```python
from build123d import *

# Parameters (mm, degrees)
SKETCH1_R            = 15
SKETCH1_R_2          = 1.25
BOSS_EXTRUDE1_DEPTH  = 1.3
FILLET1_R            = 1
SKETCH2_R            = 35.5
SKETCH2_R_2          = 0.625
BOSS_EXTRUDE2_DEPTH  = 0.1
SKETCH4_R            = 0.625
SKETCH4_R_2          = 31.5
BOSS_EXTRUDE4_DEPTH  = 0.1
SKETCH5_R            = 27.5
SKETCH5_R_2          = 0.625
BOSS_EXTRUDE5_DEPTH  = 0.1
SKETCH6_R            = 23.5
SKETCH6_R_2          = 0.625
BOSS_EXTRUDE6_DEPTH  = 0.1
SKETCH7_R            = 19.5
SKETCH7_R_2          = 0.625
BOSS_EXTRUDE7_DEPTH  = 0.1
SKETCH8_R            = 15.5
SKETCH8_R_2          = 0.625
BOSS_EXTRUDE8_DEPTH  = 0.1
BOSS_EXTRUDE9_DEPTH  = 0.1
BOSS_EXTRUDE10_DEPTH = 0.1
BOSS_EXTRUDE11_DEPTH = 0.1
BOSS_EXTRUDE12_DEPTH = 0.1
BOSS_EXTRUDE13_DEPTH = 0.1
BOSS_EXTRUDE14_DEPTH = 0.1
CUT_EXTRUDE1_START   = -1.5
SKETCH10_R           = 0.625
CUT_EXTRUDE1_DEPTH   = 1.5


with BuildPart() as part:
    # Sketch1 → Boss-Extrude1 (new body)
    with BuildSketch(Plane(origin=(0, 0, 0), x_dir=(1, 0, 0), z_dir=(0, 1, 0))):
        with BuildLine():
            ThreePointArc((-40, 0), (-29.325037044, -27.203716701), (-2.997889883, -39.8875))
            ThreePointArc((-2.997889883, -39.8875), (0, -43), (2.997889883, -39.8875))
            ThreePointArc((2.997889883, -39.8875), (40, 0), (2.997889883, 39.8875))
            ThreePointArc((2.997889883, 39.8875), (0, 43), (-2.997889883, 39.8875))
            ThreePointArc((-2.997889883, 39.8875), (-29.325037044, 27.203716701), (-40, 0))
        make_face()
        with Locations(Location((0, 0, 0), (0, 0, 270))):
            Circle(SKETCH1_R, mode=Mode.SUBTRACT)
        with Locations(Location((0, 40, 0), (0, 0, 270))):
            Circle(SKETCH1_R_2, mode=Mode.SUBTRACT)
        with Locations(Location((0, -40, 0), (0, 0, 270))):
            Circle(SKETCH1_R_2, mode=Mode.SUBTRACT)
    extrude(amount=BOSS_EXTRUDE1_DEPTH)

    # Fillet1
    fillet1_edges = [part.edges().sort_by_distance(p)[0] for p in [
        (-2.997889883, 0.65, -39.8875),
        (2.997889883, 0.65, -39.8875),
        (2.997889883, 0.65, 39.8875),
        (-2.997889883, 0.65, 39.8875),
    ]]
    fillet(fillet1_edges, radius=FILLET1_R)

    # Sketch2 → Boss-Extrude2 (add)
    with BuildSketch(Plane(origin=(0, 1.3, 0), x_dir=(1, 0, 0), z_dir=(0, 1, 0))):
        with BuildLine():
            ThreePointArc((37.47, 1.49969997), (-37.5, 0), (37.47, -1.49969997))
            ThreePointArc((37.47, -1.49969997), (39, 0), (37.47, 1.49969997))
        make_face()
        with Locations(Location((0, 0, 0), (0, 0, 270))):
            Circle(SKETCH2_R, mode=Mode.SUBTRACT)
        with Locations(Location((38.25, 0, 0), (0, 0, 270))):
            Circle(SKETCH2_R_2, mode=Mode.SUBTRACT)
    extrude(amount=BOSS_EXTRUDE2_DEPTH)

    # Sketch4 → Boss-Extrude4 (add)
    with BuildSketch(Plane(origin=(0, 1.3, 0), x_dir=(1, 0, 0), z_dir=(0, 1, 0))):
        with BuildLine():
            ThreePointArc((33.46641791, -1.499624034), (35, 0), (33.46641791, 1.499624034))
            ThreePointArc((33.46641791, 1.499624034), (-33.5, 0), (33.46641791, -1.499624034))
        make_face()
        with Locations(Location((34.25, 0, 0), (0, 0, 270))):
            Circle(SKETCH4_R, mode=Mode.SUBTRACT)
        with Locations(Location((0, 0, 0), (0, 0, 270))):
            Circle(SKETCH4_R_2, mode=Mode.SUBTRACT)
    extrude(amount=BOSS_EXTRUDE4_DEPTH)

    # Sketch5 → Boss-Extrude5 (add)
    with BuildSketch(Plane(origin=(0, 1.3, 0), x_dir=(1, 0, 0), z_dir=(0, 1, 0))):
        with BuildLine():
            ThreePointArc((29.461864407, 1.499515147), (-29.5, 0), (29.461864407, -1.499515147))
            ThreePointArc((29.461864407, -1.499515147), (31, 0), (29.461864407, 1.499515147))
        make_face()
        with Locations(Location((0, 0, 0), (0, 0, 270))):
            Circle(SKETCH5_R, mode=Mode.SUBTRACT)
        with Locations(Location((30.25, 0, 0), (0, 0, 270))):
            Circle(SKETCH5_R_2, mode=Mode.SUBTRACT)
    extrude(amount=BOSS_EXTRUDE5_DEPTH)

    # Sketch6 → Boss-Extrude6 (add)
    with BuildSketch(Plane(origin=(0, 1.3, 0), x_dir=(1, 0, 0), z_dir=(0, 1, 0))):
        with BuildLine():
            ThreePointArc((25.455882353, 1.499351071), (-25.5, 0), (25.455882353, -1.499351071))
            ThreePointArc((25.455882353, -1.499351071), (27, 0), (25.455882353, 1.499351071))
        make_face()
        with Locations(Location((0, 0, 0), (0, 0, 270))):
            Circle(SKETCH6_R, mode=Mode.SUBTRACT)
        with Locations(Location((26.25, 0, 0), (0, 0, 270))):
            Circle(SKETCH6_R_2, mode=Mode.SUBTRACT)
    extrude(amount=BOSS_EXTRUDE6_DEPTH)

    # Sketch7 → Boss-Extrude7 (add)
    with BuildSketch(Plane(origin=(0, 1.3, 0), x_dir=(1, 0, 0), z_dir=(0, 1, 0))):
        with BuildLine():
            ThreePointArc((21.447674419, 1.499087067), (-21.5, 0), (21.447674419, -1.499087067))
            ThreePointArc((21.447674419, -1.499087067), (23, 0), (21.447674419, 1.499087067))
        make_face()
        with Locations(Location((0, 0, 0), (0, 0, 270))):
            Circle(SKETCH7_R, mode=Mode.SUBTRACT)
        with Locations(Location((22.25, 0, 0), (0, 0, 270))):
            Circle(SKETCH7_R_2, mode=Mode.SUBTRACT)
    extrude(amount=BOSS_EXTRUDE7_DEPTH)

    # Sketch8 → Boss-Extrude8 (add)
    with BuildSketch(Plane(origin=(0, 1.3, 0), x_dir=(1, 0, 0), z_dir=(0, 1, 0))):
        with BuildLine():
            ThreePointArc((17.435714286, 1.498621816), (-17.5, 0), (17.435714286, -1.498621816))
            ThreePointArc((17.435714286, -1.498621816), (19, 0), (17.435714286, 1.498621816))
        make_face()
        with Locations(Location((0, 0, 0), (0, 0, 270))):
            Circle(SKETCH8_R, mode=Mode.SUBTRACT)
        with Locations(Location((18.25, 0, 0), (0, 0, 270))):
            Circle(SKETCH8_R_2, mode=Mode.SUBTRACT)
    extrude(amount=BOSS_EXTRUDE8_DEPTH)

    # Sketch12 → Boss-Extrude9 (add)
    with BuildSketch(Plane.XZ):
        with BuildLine():
            Line((3.725557051, 38.821646341), (3.510621067, 36.581935976))
            ThreePointArc((3.510621067, 36.581935976), (36.75, 0), (3.510621067, -36.581935976))
            Line((3.510621067, -36.581935976), (3.725557051, -38.821646341))
            ThreePointArc((3.725557051, -38.821646341), (39, 0), (3.725557051, 38.821646341))
        make_face()
    extrude(amount=BOSS_EXTRUDE9_DEPTH)

    # Sketch13 → Boss-Extrude10 (add)
    with BuildSketch(Plane.XZ):
        with BuildLine():
            Line((3.367330411, 35.088795732), (3.128512652, 32.600228659))
            ThreePointArc((3.128512652, 32.600228659), (32.75, 0), (3.128512652, -32.600228659))
            Line((3.128512652, -32.600228659), (3.367330411, -35.088795732))
            ThreePointArc((3.367330411, -35.088795732), (35.25, 0), (3.367330411, 35.088795732))
        make_face()
    extrude(amount=BOSS_EXTRUDE10_DEPTH)

    # Sketch14 → Boss-Extrude11 (add)
    with BuildSketch(Plane.XZ):
        with BuildLine():
            Line((2.985221996, 31.107088415), (2.746404236, 28.618521341))
            ThreePointArc((2.746404236, 28.618521341), (28.75, 0), (2.746404236, -28.618521341))
            Line((2.746404236, -28.618521341), (2.985221996, -31.107088415))
            ThreePointArc((2.985221996, -31.107088415), (31.25, 0), (2.985221996, 31.107088415))
        make_face()
    extrude(amount=BOSS_EXTRUDE11_DEPTH)

    # Sketch15 → Boss-Extrude12 (add)
    with BuildSketch(Plane.XZ):
        with BuildLine():
            Line((2.60311358, 27.125381098), (2.364295821, 24.636814024))
            ThreePointArc((2.364295821, 24.636814024), (24.75, 0), (2.364295821, -24.636814024))
            Line((2.364295821, -24.636814024), (2.60311358, -27.125381098))
            ThreePointArc((2.60311358, -27.125381098), (27.25, 0), (2.60311358, 27.125381098))
        make_face()
    extrude(amount=BOSS_EXTRUDE12_DEPTH)

    # Sketch16 → Boss-Extrude13 (add)
    with BuildSketch(Plane.XZ):
        with BuildLine():
            Line((1.982187405, 20.655106707), (2.221005165, 23.14367378))
            ThreePointArc((2.221005165, 23.14367378), (23.25, 0), (2.221005165, -23.14367378))
            Line((2.221005165, -23.14367378), (1.982187405, -20.655106707))
            ThreePointArc((1.982187405, -20.655106707), (20.75, 0), (1.982187405, 20.655106707))
        make_face()
    extrude(amount=BOSS_EXTRUDE13_DEPTH)

    # Sketch17 → Boss-Extrude14 (add)
    with BuildSketch(Plane.XZ):
        with BuildLine():
            Line((1.838896749, 19.161966463), (1.60007899, 16.67339939))
            ThreePointArc((1.60007899, 16.67339939), (16.75, 0), (1.60007899, -16.67339939))
            Line((1.60007899, -16.67339939), (1.838896749, -19.161966463))
            ThreePointArc((1.838896749, -19.161966463), (19.25, 0), (1.838896749, 19.161966463))
        make_face()
    extrude(amount=BOSS_EXTRUDE14_DEPTH)

    # Sketch10 → Cut-Extrude1 (cut)
    with BuildSketch(Plane(origin=(0, 1.3, 0), x_dir=(1, 0, 0), z_dir=(0, 1, 0)).offset(CUT_EXTRUDE1_START)):
        with Locations(Location((38.25, 0, 0), (0, 0, 90))):
            Circle(SKETCH10_R)
        with Locations(Location((34.25, 0, 0), (0, 0, 90))):
            Circle(SKETCH10_R)
        with Locations(Location((30.25, 0, 0), (0, 0, 90))):
            Circle(SKETCH10_R)
        with Locations(Location((26.25, 0, 0), (0, 0, 90))):
            Circle(SKETCH10_R)
        with Locations(Location((22.25, 0, 0), (0, 0, 90))):
            Circle(SKETCH10_R)
        with Locations(Location((18.25, 0, 0), (0, 0, 90))):
            Circle(SKETCH10_R)
    extrude(amount=CUT_EXTRUDE1_DEPTH, mode=Mode.SUBTRACT)


solid = part.part
```
Source: CAD feature listing. Evaluate the final solid. Frame: model axes, mm. A direction names the side the tool comes from. Give positions to 0.01 mm unless a question says otherwise; leave off trailing zeros. Use a Markdown table: item, result. Add a question column.
(1) Section query A-A (y = 0.45). Count the separate pieces of the cut face and the enclosed holes in it, then the cut area to 3 significant figures.
(2) Pull-direction query (X, two-part tool) for faces 3 (the face through (-23, 1.3, 12)), 4 (the face through (21, -0.1, -5)), 5 (the face through (0, 1, -43)); classes: +X half, -X half, draft (parallel to the pull), parting line (faces both ways), or undercut.
(3) Ray query, line 1 (Z direction, x = -6, y = 0.25); line 2 (Y direction, x = -33.5, z = -11.5); line 3 (X direction, y = 0.55, z = 40). Return the intervals inside material, ascending.
(4) Access query for faces 1 (the face through (-21.203, 1.3, 26.131)), 2 (the face through (29, -0.1, -4)). Directions: +Z, -Z, +X, -X, +Y, -Y. A direction counts if a zero-diameter tool reaches every point of the face in a straight line with its end or side. Return the directions, or none.
(5) First-contact query: pin 1 Ø25 at (x, z) = (0, 0) entering from +Y; pin 2 Ø2 at (x, z) = (-30, 12.5) entering from -Y. Flat tips, straight axial feed; report the tip coordinate or a pass-through.
Checked values:
| question | item | result |
|---|---|---|
| 1 | separate pieces | 1 |
| 1 | enclosed holes | 9 |
| 1 | area | 4,330 mm^2 |
| 2 | face 3 | undercut |
| 2 | face 4 | draft |
| 2 | face 5 | parting line |
| 3 | line 1 | -39.55 to -13.75, 13.75 to 39.55 |
| 3 | line 2 | 0 to 1.3 |
| 3 | line 3 | -3.33 to -1.25, 1.25 to 3.33 |
| 4 | face 1 | +Y |
| 4 | face 2 | +Z, -Z, +X, -X, -Y |
| 5 | pin 1 | through |
| 5 | pin 2 | y = 0 |
